Geometry check sheet. Reference: the model listing, model coordinates, mm. A direction names the side the tool comes from. Give positions to 0.01 mm unless a question says otherwise; leave off trailing zeros. Write each loop counter-clockwise with the first axis right and the second up, starting at its lowest first coordinate (ties: lowest second). Pieces come first, ordered by that corner, then holes. Notation, with made-up numbers: (-14.75, 10.25) -> (40.25, 10.25) arc R35 cw to (40.25, 44.25) -> close; hole circle Ø5 at (-37.75, 4.5). An arc over 180 degrees is marked (long way). Write item = value, one per line. Start each with the question number.
1. Cross-section at D-D, the plane y = 9. Record the cut outline in (x, z), plus the area to 3 significant figures.
2. Thickness scan on line 1 along Y through (x, z) = (0, 3); line 2 along X through (y, z) = (-8.4, 0); line 3 along Y through (x, z) = (4.25, -3.5). Record the ranges inside material, lowest first.
3. Cross-section at B-B, the plane y = 0. Record the cut outline in (x, z).
4. Depth check by flat-ended pin: P1, Ø3, axis at y = -3, z = -4.5, coming from the -X side; P2, Ø2, axis at x = -1, z = -6, coming from the +Y side; P3, Ø2.5, axis at x = 0, z = 0, coming from the -Y side. Enter the tip coordinate at first touch or a pass-through.
5. Cross-section at C-C, the plane x = 0. Record the cut outline in (y, z), plus the area to 3 significant figures.
6. Set-up check for faces 5 (the cylindrical face through (9, -12, 0)), 6 (the flat face through (2, 10, -2)), 7 (the flat face through (-3.5, -6.5, -8)): record each of +Z, -Z, +X, -X, +Y, -Y from which the full face is reachable in a straight line by a thin tool's end or side.
7. Mould release check, pull along Z, two halves, no side actions. Record for faces 1 (the flat face through (-10, -15, 0)), 2 (the flat face through (-3.5, -6.5, 8)), 3 (the cylindrical face through (-11, 0, 0)), 4 (the flat face through (2, -10, 2)): pulls with the +Z half, pulls with the -Z half, needs draft (parallel to the pull), parting line crosses it, or undercut.
8. Cross-section at A-A, the plane z = 0. Record the cut outline in (x, y), plus the area to 3 significant figures.
```python
from build123d import *

# Parameters (mm, degrees)
ESQUISSE2_W             = 4
ESQUISSE2_H             = 32
ENL_V_MAT_EXTRU_1_DEPTH = 42.194659848
ESQUISSE3_R             = 7
ENL_V_MAT_EXTRU_2_DEPTH = 25.535688419


with BuildPart() as part:
    # Esquisse1 → Base-Révolution (revolve)
    with BuildSketch(Plane.XY, mode=Mode.PRIVATE) as base_r_volution_sk:
        with BuildLine():
            Line((-2, 10), (-8.5, 10))
            ThreePointArc((-8.5, 10), (-8.853553391, 10.146446609), (-9, 10.5))
            Line((-9, 10.5), (-9, 14.5))
            ThreePointArc((-9, 14.5), (-9.146446609, 14.853553391), (-9.5, 15))
            Line((-9.5, 15), (-11, 15))
            Line((-11, 15), (-11, -15))
            Line((-11, -15), (-9.5, -15))
            ThreePointArc((-9.5, -15), (-9.146446609, -14.853553391), (-9, -14.5))
            Line((-9, -14.5), (-9, -10.5))
            ThreePointArc((-9, -10.5), (-8.853553391, -10.146446609), (-8.5, -10))
            Line((-8.5, -10), (-2, -10))
            Line((-2, -10), (-2, 10))
        make_face()
    revolve(base_r_volution_sk.sketch.rotate(Axis((0, 0, 0), (0, -1, 0)), 270), axis=Axis((0, 0, 0), (0, -1, 0)))

    # Esquisse2 → Enlèv. mat.-Extru.1 (cut, through all)
    with BuildSketch(Plane(origin=(-15, 15, 0), x_dir=(0, 0, -1), z_dir=(0, -1, 0))):
        with Locations((10, 11.76635514)):
            Rectangle(ESQUISSE2_W, ESQUISSE2_H)
        with Locations((-10, 11.76635514)):
            Rectangle(ESQUISSE2_W, ESQUISSE2_H)
    extrude(amount=ENL_V_MAT_EXTRU_1_DEPTH, mode=Mode.SUBTRACT)

    # Esquisse3 → Enlèv. mat.-Extru.2 (cut, through all)
    with BuildSketch(Plane.XY.offset(8)):
        Circle(ESQUISSE3_R)
    extrude(amount=-ENL_V_MAT_EXTRU_2_DEPTH, mode=Mode.SUBTRACT)


solid = part.part
```
Answers:
q1.outline = (-7.55, -8) -> (7.55, -8) arc R11 ccw to (7.55, 8) -> (-7.55, 8) arc R11 ccw to start; hole circle Ø4 at (0, 0)
q1.area = 305 mm^2
q2.line_1 = -10 to -7, 7 to 10
q2.line_2 = -11 to -2, 2 to 11
q2.line_3 = -10 to -5.56, 5.56 to 10
q3.outline = (-7.55, -8) -> (-7, -8) -> (-7, 8) -> (-7.55, 8) arc R11 ccw to start; (7, -8) -> (7.55, -8) arc R11 ccw to (7.55, 8) -> (7, 8) -> close
q4.P1 = -10.58
q4.P2 = 10
q4.P3 = through
q5.outline = (-10, -8) -> (-7, -8) -> (-7, -2) -> (-10, -2) -> close; (-10, 2) -> (-7, 2) -> (-7, 8) -> (-10, 8) -> close; (7, -8) -> (10, -8) -> (10, -2) -> (7, -2) -> close; (7, 2) -> (10, 2) -> (10, 8) -> (7, 8) -> close
q5.area = 72.0 mm^2
q6.face_5 = -Y
q6.face_6 = +Y
q6.face_7 = -Z, +X, -X, +Y, -Y
q7.face_1 = needs draft
q7.face_2 = pulls with the +Z half
q7.face_3 = parting line crosses it
q7.face_4 = undercut
q8.outline = (-11, -15) -> (-9.5, -15) arc R0.5 ccw to (-9, -14.5) -> (-9, -10.5) arc R0.5 cw to (-8.5, -10) -> (-2, -10) -> (-2, -6.71) arc R7 cw to (-2, 6.71) -> (-2, 10) -> (-8.5, 10) arc R0.5 cw to (-9, 10.5) -> (-9, 14.5) arc R0.5 ccw to (-9.5, 15) -> (-11, 15) -> close; (2, -10) -> (8.5, -10) arc R0.5 cw to (9, -10.5) -> (9, -14.5) arc R0.5 ccw to (9.5, -15) -> (11, -15) -> (11, 15) -> (9.5, 15) arc R0.5 ccw to (9, 14.5) -> (9, 10.5) arc R0.5 cw to (8.5, 10) -> (2, 10) -> (2, 6.71) arc R7 cw to (2, -6.71) -> close
q8.area = 301 mm^2
